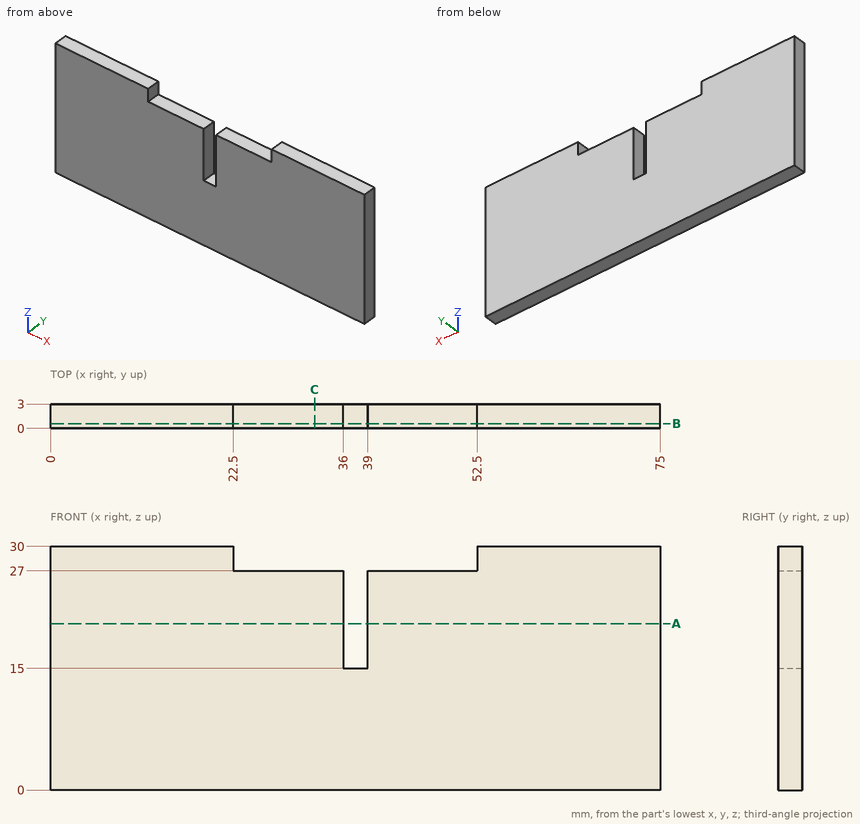
Drawing for the job (mm, zero at the part's lowest x, y, z). Round coordinates to 2 decimals unless told otherwise and drop trailing zeros. Write each loop counter-clockwise with the first axis right and the second up, starting at its lowest first coordinate (ties: lowest second). Pieces come first, ordered by that corner, then holes. Notation, with made-up numbers: (7, -16) - (59, -16) arc R26 ccw to (59, 4) - close; hole circle Ø3 at (-3, 81). An arc over 180 degrees is marked (long way). Write item = value, one per line. Start each with the question number.
Q1. Band-saw the part on C-C (x = 32.5). Give the cut face in (y, z).
Q2. Drop a flat-ended pin along its axis: pin 1 (1.5 mm diameter, centred on x = 37.5, y = 1.5, fed in from +Z). Give the stop position or say it passes through.
Q3. Band-saw the part on B-B (y = 0.6). Give the cut face in (x, z).
Q4. Band-saw the part on A-A (z = 20.5). Give the cut face in (x, y).
Q5. Probe L1, parallel to X at y = 2.35, z = 18; L2, parallel to X at y = 1.8, z = 28.25; L3, parallel to Z at x = 52, y = 0.8. List the from-to ranges inside material, lowest first. Write a range as from..to.
Answers below:
q1.outline = (0, 0) - (3, 0) - (3, 27) - (0, 27) - close
q2.pin_1 = 15
q3.outline = (0, 0) - (75, 0) - (75, 30) - (52.5, 30) - (52.5, 27) - (39, 27) - (39, 15) - (36, 15) - (36, 27) - (22.5, 27) - (22.5, 30) - (0, 30) - close
q4.outline = (0, 0) - (36, 0) - (36, 3) - (0, 3) - close; (39, 0) - (75, 0) - (75, 3) - (39, 3) - close
q5.L1 = 0..36, 39..75
q5.L2 = 0..22.5, 52.5..75
q5.L3 = 0..27
